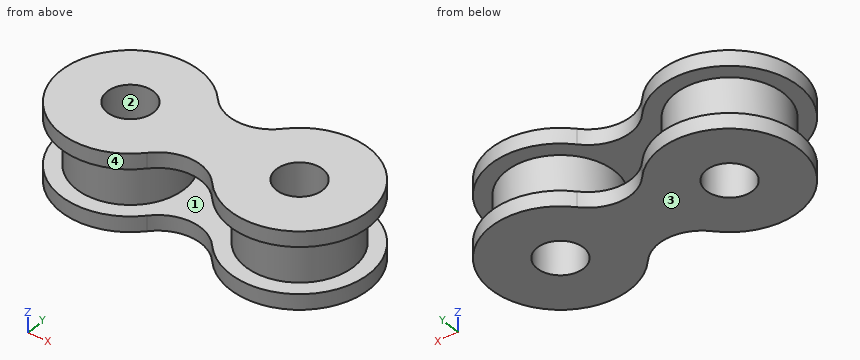
from build123d import *

# Parameters (mm, degrees)
CROQUIS1_R              = 1.5
SALIENTE_EXTRUIR1_DEPTH = 1
CROQUIS2_R              = 3.5
CROQUIS2_R_2            = 1.5
SALIENTE_EXTRUIR2_DEPTH = 3
CROQUIS3_R              = 1.5
SALIENTE_EXTRUIR3_DEPTH = 1


with BuildPart() as part:
    # Croquis1 → Saliente-Extruir1 (new body)
    with BuildSketch(Plane.XY):
        with BuildLine():
            ThreePointArc((2.109589041, -2.95890411), (10, 0), (2.109589041, 2.95890411))
            ThreePointArc((2.109589041, 2.95890411), (0, 2), (-2.109589041, 2.95890411))
            ThreePointArc((-2.109589041, 2.95890411), (-10, 0), (-2.109589041, -2.95890411))
            ThreePointArc((-2.109589041, -2.95890411), (0, -2), (2.109589041, -2.95890411))
        make_face()
        with Locations((-5.5, 0)):
            Circle(CROQUIS1_R, mode=Mode.SUBTRACT)
        with Locations((5.5, 0)):
            Circle(CROQUIS1_R, mode=Mode.SUBTRACT)
    extrude(amount=SALIENTE_EXTRUIR1_DEPTH)

    # Croquis2 → Saliente-Extruir2 (add)
    with BuildSketch(Plane.XY.offset(1)):
        with Locations((-5.5, 0)):
            Circle(CROQUIS2_R)
        with Locations((-5.5, 0)):
            Circle(CROQUIS2_R_2, mode=Mode.SUBTRACT)
        with Locations((5.5, 0)):
            Circle(CROQUIS2_R)
        with Locations((5.5, 0)):
            Circle(CROQUIS2_R_2, mode=Mode.SUBTRACT)
    extrude(amount=SALIENTE_EXTRUIR2_DEPTH)

    # Croquis3 → Saliente-Extruir3 (add)
    with BuildSketch(Plane.XY.offset(4)):
        with BuildLine():
            ThreePointArc((-2.109589041, 2.95890411), (0, 2), (2.109589041, 2.95890411))
            ThreePointArc((2.109589041, 2.95890411), (10, 0), (2.109589041, -2.95890411))
            ThreePointArc((2.109589041, -2.95890411), (0, -2), (-2.109589041, -2.95890411))
            ThreePointArc((-2.109589041, -2.95890411), (-10, 0), (-2.109589041, 2.95890411))
        make_face()
        with Locations((-5.5, 0)):
            Circle(CROQUIS3_R, mode=Mode.SUBTRACT)
        with Locations((5.5, 0)):
            Circle(CROQUIS3_R, mode=Mode.SUBTRACT)
    extrude(amount=SALIENTE_EXTRUIR3_DEPTH)


solid = part.part
Check sheet for the modelled part. Datum: model origin and axes. Units: mm. Face numbers are marked on the shaded views. A direction names the side the tool comes from. Round coordinates to 2 decimals unless told otherwise and drop trailing zeros. Order: outer loops, then holes, each group sorted by start corner. A loop starts at its lowest first (then second) coordinate and runs counter-clockwise, first axis right, second up. Notation, with made-up numbers: M 9,59 L 50,59 A30 cw 50,90 Z; hole C 82,52.25 d4. An arc over 180 degrees is marked long. One line per item, written item: value. Start each with the question number.
1. Section check A-A on y = 0. Enter the section's corners in (x, z).
2. Gauge pin test, flat end, axial feed: P1, Ø2.5, axis at x = -5.5, y = 0, coming from the -Z side. Record the tip position at first contact, or that the pin passes through.
3. Access from +Z, -Z, +X, -X, +Y, -Y to the whole of each face (thin tool, end or side, straight path). Record for the marked faces 1 and 2.
4. Section check C-C on x = -5.5. Enter the section's corners in (y, z), and give its area (3 significant figures).
5. Scan lines: line 1 along Y through (x, z) = (5.5, 1.6); line 2 along Z through (x, y) = (0.5, 1); line 3 along X through (y, z) = (-2, 1.9). Record each from-to range of solid material in increasing order.
6. Section check B-B on z = 1.95. Enter the section's corners in (x, y).
7. Section check D-D on z = 0.4. Enter the section's corners in (x, y), and give its area (3 significant figures).
8. Release check for a two-part mould opening along X. For the marked faces 3 and 4 record: released by +X, released by -X, zero draft, split by the parting line, or undercut.
Results found:
1. outline: M -10,0 L -7,0 L -7,5 L -10,5 L -10,4 L -9,4 L -9,1 L -10,1 Z; M -4,0 L 4,0 L 4,5 L -4,5 Z; M 7,0 L 10,0 L 10,1 L 9,1 L 9,4 L 10,4 L 10,5 L 7,5 Z; hole M -2,1 L 2,1 L 2,4 L -2,4 Z
2. P1: through
3. face 1: none
3. face 2: +Z, -Z
4. outline: M -4.5,0 L -1.5,0 L -1.5,5 L -4.5,5 L -4.5,4 L -3.5,4 L -3.5,1 L -4.5,1 Z; M 1.5,0 L 4.5,0 L 4.5,1 L 3.5,1 L 3.5,4 L 4.5,4 L 4.5,5 L 1.5,5 Z
4. area: 24.0 mm^2
5. line 1: -3.5 to -1.5, 1.5 to 3.5
5. line 2: 0 to 1, 4 to 5
5. line 3: -8.37 to -2.63, 2.63 to 8.37
6. outline: C -5.5,0 d7; C 5.5,0 d7; hole C -5.5,0 d3; hole C 5.5,0 d3
7. outline: M -2.11,-2.96 A2.8 cw 2.11,-2.96 A4.5 ccw long 2.11,2.96 A2.8 cw -2.11,2.96 A4.5 ccw long Z; hole C -5.5,0 d3; hole C 5.5,0 d3
7. area: 123 mm^2
8. face 3: zero draft
8. face 4: undercut
